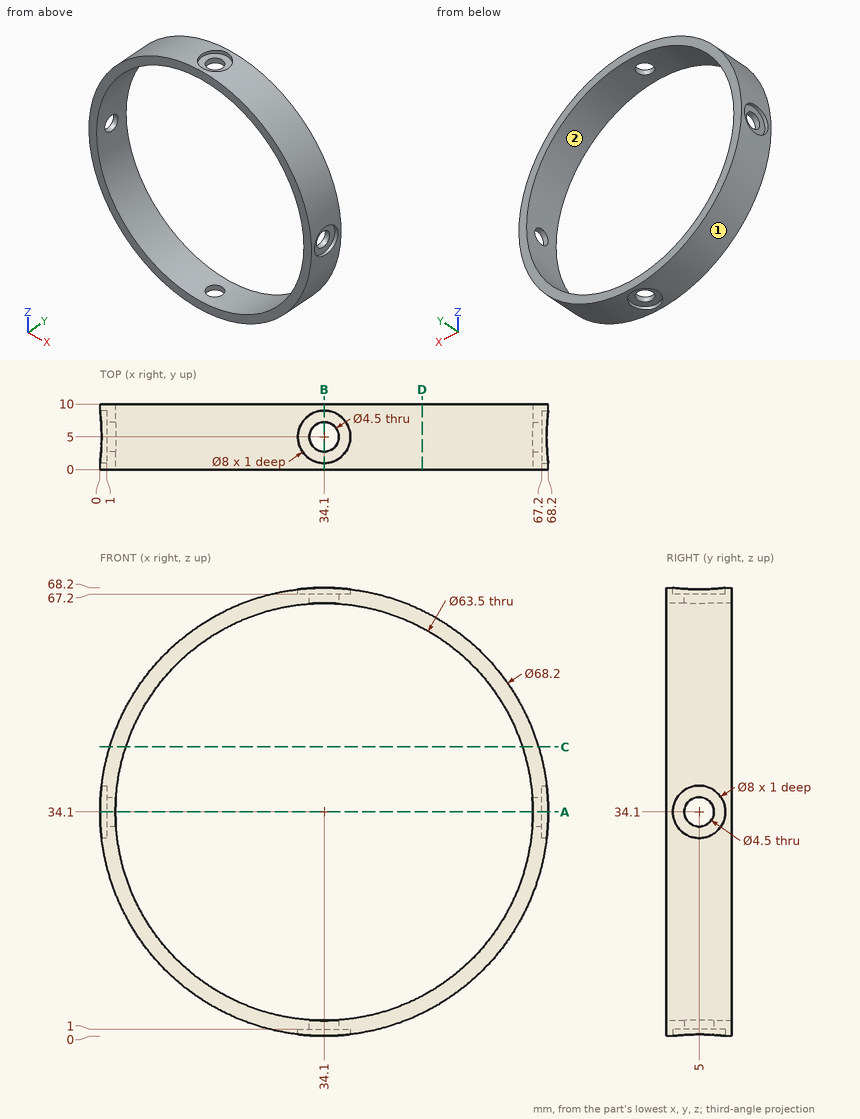
Geometry: see drawing. Coordinates: mm, zero at the bounding-box minimum. Round coordinates to 2 decimals unless told otherwise and drop trailing zeros. Write each loop counter-clockwise with the first axis right and the second up, starting at its lowest first coordinate (ties: lowest second). Pieces come first, ordered by that corner, then holes.
Item 1: Material intervals for L1, parallel to Y at x = 34, z = 2; L2, parallel to X at y = 7.5, z = 61.5; L3, parallel to Y at x = 67.95, z = 34.1, sorted ascending.
Item 2: Section query D-D (x = 49). Return loops of the section in (y, z).
Item 3: Section query C-C (z = 44). Return loops of the section in (x, y), plus the area to 3 significant figures.
Item 4: Section query A-A (z = 34.1). Return loops of the section in (x, y), plus the area to 4 significant figures.
Item 5: Mould query, pull axis X, two halves, no side actions, for the marked faces 1 and 2. Classes: +X half, -X half, draft (parallel to the pull), parting line (faces both ways), or undercut.
Item 6: Pin query (flat end, axial travel): P1, Ø1, axis at y = 1, z = 36.5, coming from the -X side; P2, Ø2.5, axis at x = 32, y = 5, coming from the +Z side; P3, Ø2, axis at y = 5, z = 18, coming from the -X side. Return the tip coordinate at first contact, or that it passes through.
Item 7: Section query B-B (x = 34.1). Return loops of the section in (y, z).
Completed:
1. L1: y = 0 to 2.75, 7.25 to 10
1. L2: x = 13.8 to 18.06, 50.14 to 54.4
1. L3: y = 0 to 1, 9 to 10
2. outline: (0, 3.43) - (10, 3.43) - (10, 6.06) - (0, 6.06) - close; (0, 62.14) - (10, 62.14) - (10, 64.77) - (0, 64.77) - close
3. outline: (1.47, 0) - (3.93, 0) - (3.93, 10) - (1.47, 10) - close; (64.27, 0) - (66.73, 0) - (66.73, 10) - (64.27, 10) - close
3. area: 49.3 mm2
4. outline: (0, 0) - (2.35, 0) - (2.35, 2.75) - (1, 2.75) - (1, 1) - (0, 1) - close; (0, 9) - (1, 9) - (1, 7.25) - (2.35, 7.25) - (2.35, 10) - (0, 10) - close; (65.85, 0) - (68.2, 0) - (68.2, 1) - (67.2, 1) - (67.2, 2.75) - (65.85, 2.75) - close; (65.85, 7.25) - (67.2, 7.25) - (67.2, 9) - (68.2, 9) - (68.2, 10) - (65.85, 10) - close
4. area: 18.85 mm2
5. face 1: parting line
5. face 2: undercut
6. P1: stops at x = 0.05
6. P2: stops at z = 67.2
6. P3: stops at x = 3.53
7. outline: (0, 0) - (1, 0) - (1, 1) - (2.75, 1) - (2.75, 2.35) - (0, 2.35) - close; (0, 65.85) - (2.75, 65.85) - (2.75, 67.2) - (1, 67.2) - (1, 68.2) - (0, 68.2) - close; (7.25, 1) - (9, 1) - (9, 0) - (10, 0) - (10, 2.35) - (7.25, 2.35) - close; (7.25, 65.85) - (10, 65.85) - (10, 68.2) - (9, 68.2) - (9, 67.2) - (7.25, 67.2) - close
